Model file for the job. Use its own axes, mm. Face numbers are marked on the shaded views. Round coordinates to 2 decimals unless told otherwise and drop trailing zeros. Order: outer loops, then holes, each group sorted by start corner. A loop starts at its lowest first (then second) coordinate and runs counter-clockwise, first axis right, second up. Notation, with made-up numbers: (37, 80) -> (85, 80) arc R8 cw to (85, 95) -> close; hole circle Ø4 at (-30.5, 20.25). An arc over 180 degrees is marked (long way). Put each result on its own line as item: value. Start each with the question number.
Q1. Cut at D-D, the plane x = 882. List the corners of the cut face in (y, z).
Q2. Probe L1, parallel to X at y = 125, z = 7; L2, parallel to X at y = 71, z = 5; L3, parallel to Y at x = 518, z = 1.75. List the from-to ranges inside material, lowest first.
Q3. Cut at A-A, the plane x = 517.5. List the corners of the cut face in (y, z).
Q4. Flat gauge pins, fed straight in: P1, Ø6.5, axis at x = 659.3, y = -62.66, coming from the -Z side; P2, Ø4, axis at y = -25.5, z = 8.5, coming from the +X side; P3, Ø3.5, axis at y = -6, z = 6.5, coming from the +X side; P4, Ø5, axis at y = -35, z = 4, coming from the +X side. Where does each tip first touch, or does it go through?
Q5. Pull direction Z, two halves, no side cores. Call the marked faces 1 and 2: released by +Z, released by -Z, zero draft, split by the parting line, or undercut.
Q6. Cut at B-B, the plane z = 4. State how many separate pieces and enclosed holes the cut face has, and give its area (3 significant figures).
Q7. Cut at C-C, the plane x = 764.5. List the corners of the cut face in (y, z), and give its area (3 significant figures).
from build123d import *

# Parameters (mm, degrees)
SKETCH_1_R          = 2.75
SKETCH_1_R_2        = 17
SKETCH_1_R_3        = 20
SKETCH_1_R_4        = 3.5
SKETCH_1_R_5        = 2
SKETCH_1_W          = 20
SKETCH_1_H          = 3
SKETCH_1_W_2        = 3.160774411
SKETCH_1_H_2        = 20
SKETCH_1_W_3        = 3
SKETCH_1_H_3        = 50
EXTRUDE_1_DEPTH     = 10
EXTRUDE_3_DEPTH     = 10
SKETCH_3_R          = 2
CUT_EXTRUDE_1_DEPTH = 999.435971659


with BuildPart() as part:
    # 스케치1 → 보스-돌출1 (new body)
    with BuildSketch(Plane.XY):
        with BuildLine():
            Line((5.267585072, -97.655469737), (35.301603788, -97.655469737))
            Line((35.301603788, -97.655469737), (35.301603788, -87.655469737))
            Line((35.301603788, -87.655469737), (85.301603788, -87.655469737))
            Line((85.301603788, -87.655469737), (85.301603788, -97.655469737))
            Line((85.301603788, -97.655469737), (85.305622503, -97.655469737))
            Line((85.305622503, -97.655469737), (135.297585072, -97.655469737))
            Line((135.297585072, -97.655469737), (135.301603788, -97.655469737))
            Line((135.301603788, -97.655469737), (135.301603788, -87.655469737))
            Line((135.301603788, -87.655469737), (185.301603788, -87.655469737))
            Line((185.301603788, -87.655469737), (185.301603788, -97.655469737))
            Line((185.301603788, -97.655469737), (231.531603788, -97.655469737))
            Line((231.531603788, -97.655469737), (235.301603788, -97.655469737))
            Line((235.301603788, -97.655469737), (235.301603788, -87.655469737))
            Line((235.301603788, -87.655469737), (285.301603788, -87.655469737))
            Line((285.301603788, -87.655469737), (285.301603788, -97.655469737))
            Line((285.301603788, -97.655469737), (335.301603788, -97.655469737))
            Line((335.301603788, -97.655469737), (335.301603788, -87.655469737))
            Line((335.301603788, -87.655469737), (385.301603788, -87.655469737))
            Line((385.301603788, -87.655469737), (385.301603788, -97.655469737))
            Line((385.301603788, -97.655469737), (435.301603788, -97.655469737))
            Line((435.301603788, -97.655469737), (435.301603788, -87.655469737))
            Line((435.301603788, -87.655469737), (485.301603788, -87.655469737))
            Line((485.301603788, -87.655469737), (485.301603788, -97.655469737))
            Line((485.301603788, -97.655469737), (535.301603788, -97.655469737))
            Line((535.301603788, -97.655469737), (535.301603788, -87.655469737))
            Line((535.301603788, -87.655469737), (585.301603788, -87.655469737))
            Line((585.301603788, -87.655469737), (585.301603788, -97.655469737))
            Line((585.301603788, -97.655469737), (635.301603788, -97.655469737))
            Line((635.301603788, -97.655469737), (635.301603788, -87.655469737))
            Line((635.301603788, -87.655469737), (685.301603788, -87.655469737))
            Line((685.301603788, -87.655469737), (685.301603788, -97.655469737))
            Line((685.301603788, -97.655469737), (690.631109923, -97.655469737))
            Line((690.631109923, -97.655469737), (980.385244165, 97.7861616))
            ThreePointArc((980.385244165, 97.7861616), (983.008498199, 131.143098655), (956.214221814, 151.183893662))
            Line((956.214221814, 151.183893662), (639.593248415, 22.344530263))
            Line((639.593248415, 22.344530263), (315.301603788, 22.344530263))
            Line((315.301603788, 22.344530263), (315.301603788, 72.661637882))
            Line((315.301603788, 72.661637882), (318.301603788, 72.661637882))
            Line((318.301603788, 72.661637882), (318.301603788, 122.661637882))
            Line((318.301603788, 122.661637882), (315.301603788, 122.661637882))
            Line((315.301603788, 122.661637882), (315.301603788, 146.501001281))
            Line((315.301603788, 146.501001281), (315.301603788, 151.183893662))
            Line((315.301603788, 151.183893662), (265.299669923, 151.183893662))
            Line((265.299669923, 151.183893662), (-4.732414928, 25.58459835))
            Line((-4.732414928, 25.58459835), (-4.732414928, -7.689488453))
            Line((-4.732414928, -7.689488453), (-7.732414928, -7.689488453))
            Line((-7.732414928, -7.689488453), (-7.732414928, -47.689488453))
            Line((-7.732414928, -47.689488453), (-4.732414928, -47.689488453))
            Line((-4.732414928, -47.689488453), (-4.732414928, -87.655469737))
            Line((-4.732414928, -87.655469737), (5.267585072, -97.655469737))
        make_face()
        with Locations((2.067585072, -80.890469737)):
            Circle(SKETCH_1_R, mode=Mode.SUBTRACT)
        with Locations((2.067585072, -14.422432305)):
            Circle(SKETCH_1_R, mode=Mode.SUBTRACT)
        with Locations((68.535622503, -14.422432305)):
            Circle(SKETCH_1_R, mode=Mode.SUBTRACT)
        with Locations((68.535622503, -80.890469737)):
            Circle(SKETCH_1_R, mode=Mode.SUBTRACT)
        with Locations((35.301603788, -62.655469737)):
            Circle(SKETCH_1_R_2, mode=Mode.SUBTRACT)
        with Locations(Location((685.301603788, -62.655469737, 0), (0, 0, 180))):
            Circle(SKETCH_1_R_3, mode=Mode.SUBTRACT)
        with Locations((951.422664578, 116.845452277)):
            Circle(SKETCH_1_R_3, mode=Mode.SUBTRACT)
        with Locations((973.404213264, 130.731110971)):
            Circle(SKETCH_1_R_4, mode=Mode.SUBTRACT)
        with Locations((930.301497775, 101.683120237)):
            Circle(SKETCH_1_R_4, mode=Mode.SUBTRACT)
        with Locations((274.301603788, -62.655469737)):
            Circle(SKETCH_1_R_3, mode=Mode.SUBTRACT)
        with Locations((248.301603788, -62.655469737)):
            Circle(SKETCH_1_R_4, mode=Mode.SUBTRACT)
        with Locations((300.301603788, -62.655469737)):
            Circle(SKETCH_1_R_4, mode=Mode.SUBTRACT)
        with Locations((392.301603788, -51.655469737)):
            Circle(SKETCH_1_R_3, mode=Mode.SUBTRACT)
        with Locations((366.301603788, -51.655469737)):
            Circle(SKETCH_1_R_4, mode=Mode.SUBTRACT)
        with Locations((418.301603788, -51.655469737)):
            Circle(SKETCH_1_R_4, mode=Mode.SUBTRACT)
        with Locations(Location((543.898689933, -14.422432305, 0), (0, 0, 180))):
            Circle(SKETCH_1_R, mode=Mode.SUBTRACT)
        with Locations(Location((477.430652501, -14.422432305, 0), (0, 0, 180))):
            Circle(SKETCH_1_R, mode=Mode.SUBTRACT)
        with Locations(Location((477.430652501, -80.890469737, 0), (0, 0, 180))):
            Circle(SKETCH_1_R, mode=Mode.SUBTRACT)
        with Locations(Location((543.898689933, -80.890469737, 0), (0, 0, 180))):
            Circle(SKETCH_1_R, mode=Mode.SUBTRACT)
        with Locations(Location((510.301603788, -62.655469737, 0), (0, 0, 180))):
            Circle(SKETCH_1_R_2, mode=Mode.SUBTRACT)
        with Locations((659.301603788, -62.655469737)):
            Circle(SKETCH_1_R_4, mode=Mode.SUBTRACT)
        with Locations((711.301603788, -62.655469737)):
            Circle(SKETCH_1_R_4, mode=Mode.SUBTRACT)
        with Locations((143.301603788, -81.655469737)):
            Circle(SKETCH_1_R_5, mode=Mode.SUBTRACT)
        with Locations((177.301603788, -81.655469737)):
            Circle(SKETCH_1_R_5, mode=Mode.SUBTRACT)
        with Locations((193.301603788, -81.655469737)):
            Circle(SKETCH_1_R_5, mode=Mode.SUBTRACT)
        with Locations((227.301603788, -81.655469737)):
            Circle(SKETCH_1_R_5, mode=Mode.SUBTRACT)
        with Locations((243.301603788, -81.655469737)):
            Circle(SKETCH_1_R_5, mode=Mode.SUBTRACT)
        with Locations((293.301603788, -81.655469737)):
            Circle(SKETCH_1_R_5, mode=Mode.SUBTRACT)
        with Locations((327.301603788, -81.655469737)):
            Circle(SKETCH_1_R_5, mode=Mode.SUBTRACT)
        with Locations((343.301603788, -81.655469737)):
            Circle(SKETCH_1_R_5, mode=Mode.SUBTRACT)
        with Locations((377.301603788, -81.655469737)):
            Circle(SKETCH_1_R_5, mode=Mode.SUBTRACT)
        with Locations((393.301603788, -81.655469737)):
            Circle(SKETCH_1_R_5, mode=Mode.SUBTRACT)
        with Locations((427.301603788, -81.655469737)):
            Circle(SKETCH_1_R_5, mode=Mode.SUBTRACT)
        with Locations((443.301603788, -81.655469737)):
            Circle(SKETCH_1_R_5, mode=Mode.SUBTRACT)
        with Locations((577.301603788, -81.655469737)):
            Circle(SKETCH_1_R_5, mode=Mode.SUBTRACT)
        with Locations((97.927235117, -45.281101066)):
            Circle(SKETCH_1_R_5, mode=Mode.SUBTRACT)
        with Locations(Location((122.675972458, -45.281101066, 0), (0, 0, 180))):
            Circle(SKETCH_1_R_5, mode=Mode.SUBTRACT)
        with Locations((122.675972458, -70.029838408)):
            Circle(SKETCH_1_R_5, mode=Mode.SUBTRACT)
        with Locations(Location((97.927235117, -70.029838408, 0), (0, 0, 180))):
            Circle(SKETCH_1_R_5, mode=Mode.SUBTRACT)
        with Locations((597.927235117, -45.281101066)):
            Circle(SKETCH_1_R_5, mode=Mode.SUBTRACT)
        with Locations(Location((622.675972458, -45.281101066, 0), (0, 0, 180))):
            Circle(SKETCH_1_R_5, mode=Mode.SUBTRACT)
        with Locations((622.675972458, -70.029838408)):
            Circle(SKETCH_1_R_5, mode=Mode.SUBTRACT)
        with Locations(Location((597.927235117, -70.029838408, 0), (0, 0, 180))):
            Circle(SKETCH_1_R_5, mode=Mode.SUBTRACT)
        with Locations((8.301603788, -5.922432305)):
            Rectangle(SKETCH_1_W, SKETCH_1_H, mode=Mode.SUBTRACT)
        with Locations((55.535622503, -5.922432305)):
            Rectangle(SKETCH_1_W, SKETCH_1_H, mode=Mode.SUBTRACT)
        with Locations((77.116009709, -27.422432305)):
            Rectangle(SKETCH_1_W_2, SKETCH_1_H_2, mode=Mode.SUBTRACT)
        with Locations((77.116009709, -67.655469737)):
            Rectangle(SKETCH_1_W_2, SKETCH_1_H_2, mode=Mode.SUBTRACT)
        with Locations((316.801603788, -62.655469737)):
            Rectangle(SKETCH_1_W_3, SKETCH_1_H_3, mode=Mode.SUBTRACT)
    extrude(amount=EXTRUDE_1_DEPTH)

    # 스케치2 → 보스-돌출3 (add)
    with BuildSketch(Plane.XY.offset(10)):
        Polygon((756.214221814, 151.183893662), (756.214221814, 69.799920885), (956.214221814, 151.183893662), (956.214221814, 156.183893662), (906.214221814, 156.183893662), (906.214221814, 151.183893662), (856.214221814, 151.183893662), (856.214221814, 156.183893662), (806.214221814, 156.183893662), (806.214221814, 151.183893662), align=None)
    extrude(amount=-EXTRUDE_3_DEPTH)

    # 스케치3 → 컷-돌출1 (cut, through all)
    with BuildSketch(Plane.XY.offset(10)):
        with Locations((746.563195632, 55.162355864)):
            Circle(SKETCH_3_R)
        with Locations((752.593781974, 40.342368402)):
            Circle(SKETCH_3_R)
        with Locations((789.170659585, 72.500291597)):
            Circle(SKETCH_3_R)
        with Locations((795.201245927, 57.680304135)):
            Circle(SKETCH_3_R)
    extrude(amount=-CUT_EXTRUDE_1_DEPTH, mode=Mode.SUBTRACT)


solid = part.part
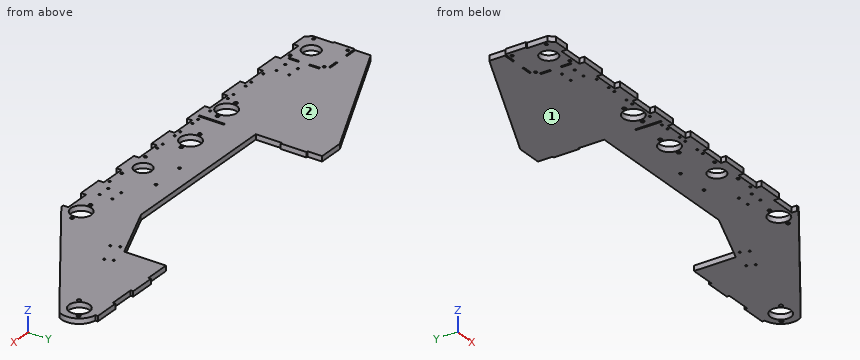
Ans:
1. outline: (31.42, 0) -> (151.18, 0) -> (151.18, 10) -> (31.42, 10) -> close
2. L1: x = 209.01 to 315.3, 756.21 to 933.16, 969.68 to 985.12
2. L2: x = 92.91 to 315.3, 756.21 to 787.85, 790.49 to 940.67
2. L3: y = -97.66 to -77.81, -47.5 to 22.34
3. outline: (-97.66, 0) -> (-78.06, 0) -> (-78.06, 10) -> (-97.66, 10) -> close; (-47.25, 0) -> (22.34, 0) -> (22.34, 10) -> (-47.25, 10) -> close
4. P1: passes through
4. P2: stops at x = 800.57
4. P3: stops at x = 829.11
4. P4: stops at x = 787.23
5. face 1: released by -Z
5. face 2: released by +Z
6. separate pieces: 1
6. enclosed holes: 52
6. area: 135,000 mm^2
7. outline: (-47.83, 0) -> (151.18, 0) -> (151.18, 10) -> (-47.83, 10) -> close
7. area: 1,990 mm^2
